Autodesk Inventor part; units mm, degrees
ref_plane "YZ Plane" through (0, 0, 0) normal (1, 0, 0) x (0, 1, 0)
ref_plane "XZ Plane" through (0, 0, 0) normal (0, 1, 0) x (-1, 0, 0)
ref_plane "XY Plane" through (0, 0, 0) normal (0, 0, 1) x (1, 0, 0)
sketch "Sketch1" plane through (0, 0, 0) normal (0, 1, 0) x (-1, 0, 0)
  circle A0 centre (0, 0) radius 30
  dimension "d0" = 60
extrude "Extrusion1" add sketch "Sketch1" along normal blind 4
sketch "Sketch2" plane through (0, 4, 0) normal (0, 1, 0) x (1, 0, 0)
  circle A0 centre (0, 0) radius 27.5
  dimension "d3" = 55
extrude "Extrusion2" add sketch "Sketch2" along normal blind 10 draft -20
sketch "Sketch3" plane through (0, 14, 0) normal (0, 1, 0) x (1, 0, 0)
  circle A0 centre (0, 0) radius 4
  dimension "d6" = 8
extrude "Extrusion3" cut sketch "Sketch3" against normal blind 16
sketch "Sketch4" plane through (0, 0, 0) normal (0, -1, 0) x (1, 0, 0)
  circle A0 centre (0, 0) radius 11
  dimension "d9" = 22
extrude "Extrusion4" cut sketch "Sketch4" against normal blind 7
sketch "Sketch5" plane through (0, 7, 0) normal (0, -1, 0) x (1, 0, 0)
  circle A0 centre (0, 0) radius 10.5
  dimension "d12" = 21
extrude "Extrusion5" cut sketch "Sketch5" against normal blind 17
properties part number "spool holder"
Input: part model. Units: mm. Frame: model coordinates. A direction names the side the tool comes from. Round coordinates to 2 decimals unless told otherwise and drop trailing zeros. Loops run counter-clockwise (first coordinate to the right, second up) from the corner with the lowest first, then second, coordinate; pieces in that order, holes last. Notation, with made-up numbers: (14.5, 76) -> (56.5, 76) arc R16 ccw to (56.5, 98) -> close; hole circle Ø1 at (29, 64.5). An arc over 180 degrees is marked (long way). Answer as a JSON object with one key per item and string values. Group by question number.
1) Ray query, L1, parallel to Z at x = 0, y = 3.5; L2, parallel to X at y = 2, z = -10; L3, parallel to X at y = 11.5, z = -6. Return the intervals inside material, ascending.
2) Section query A-A on x = 0. Output: boundary loops of the cut face in (y, z), plus the area to 3 significant figures.
3) Pin query (flat end, axial travel): pin 1 (6 mm diameter, centred on y = 12.5, z = -12.5, fed in from +X); pin 2 (10 mm diameter, centred on x = -0.5, z = 3, fed in from -Y); pin 3 (6 mm diameter, centred on y = 8, z = 17.5, fed in from -X); pin 4 (1 mm diameter, centred on x = 3.5, y = 7.5, fed in from -Z). Return the tip coordinate at first contact, or that it passes through.
4) Draft query along Z for faces 1 (the flat face through (0, 0, -13)), 2 (the cylindrical face through (10, 10.5, 3.2)), 3 (the flat face through (10, 7, -4)), 4 (the cylindrical face through (29.97, 1.97, -1.32)). Return one class per face: +Z half, -Z half, draft (parallel to the pull), parting line (faces both ways), or undercut.
5) Section query C-C on y = 2. Output: boundary loops of the cut face in (x, z).
6) Section query B-B on z = 0. Output: boundary loops of the cut face in (x, y).
7) Reachability of faces 5 (the flat face through (-13.2, 4, -24.3)), 6 (the flat face through (10, 14, 5)), 7 (the cylindrical face through (-2.38, 3.45, -10.74)) from +Z, -Z, +X, -X, +Y, -Y: full face, straight path, thin tool, end or side. Return the list, or none.
8) Section query D-D on y = 6. Output: boundary loops of the cut face in (x, z).
Reply:
{
 "1": {"L1": "z = -30 to -11, 11 to 30", "L2": "x = -28.28 to -4.58, 4.58 to 28.28", "L3": "x = -24.03 to -8.62, 8.62 to 24.03"},
 "2": {"outline": "(0, -30) -> (4, -30) -> (4, -27.5) -> (14, -23.86) -> (14, -10.5) -> (7, -10.5) -> (7, -11) -> (0, -11) -> close; (0, 11) -> (7, 11) -> (7, 10.5) -> (14, 10.5) -> (14, 23.86) -> (4, 27.5) -> (4, 30) -> (0, 30) -> close", "area": "453 mm2"},
 "3": {"pin 1": "stops at x = 22.94", "pin 2": "passes through", "pin 3": "stops at x = -22.03", "pin 4": "stops at z = -26.19"},
 "4": {"face 1": "draft", "face 2": "undercut", "face 3": "undercut", "face 4": "parting line"},
 "5": {"outline": "circle Ø60 at (0, 0); hole circle Ø22 at (0, 0)"},
 "6": {"outline": "(-30, 0) -> (-11, 0) -> (-11, 7) -> (-10.5, 7) -> (-10.5, 14) -> (-23.86, 14) -> (-27.5, 4) -> (-30, 4) -> close; (10.5, 7) -> (11, 7) -> (11, 0) -> (30, 0) -> (30, 4) -> (27.5, 4) -> (23.86, 14) -> (10.5, 14) -> close"},
 "7": {"face 5": "+Y", "face 6": "+Z, -Z, +X, -X, +Y", "face 7": "-Y"},
 "8": {"outline": "circle Ø53.54 at (0, 0); hole circle Ø22 at (0, 0)"}
}
